```python
from build123d import *

# Parameters (mm, degrees)
F0_W     = 140
F0_H     = 60
F1_DEPTH = 60
F2_R     = 10
F5_DEPTH = 10
F4_R     = 10
F6_DEPTH = 103.2
F3_R     = 10
F7_DEPTH = 10
F8_R     = 5


with BuildPart() as f1:
    # F0 (on Top) → F1 (new body)
    with BuildSketch(Plane.XY):
        Rectangle(F0_W, F0_H)
    extrude(amount=F1_DEPTH)

    # F2 (on face) → F5 (join)
    with BuildSketch(Plane.XY.offset(60)):
        with Locations((-40, 0)):
            Circle(F2_R)
    extrude(amount=F5_DEPTH)

    # F4 (on face) → F6 (cut)
    with BuildSketch(Plane.XY.offset(60)):
        Circle(F4_R)
    extrude(amount=-F6_DEPTH, mode=Mode.SUBTRACT)

    # F3 (on face) → F7 (cut)
    with BuildSketch(Plane.XY.offset(60)):
        with Locations((40, 0)):
            Circle(F3_R)
    extrude(amount=-F7_DEPTH, mode=Mode.SUBTRACT)

    # F8
    f8_edges = [f1.edges().sort_by_distance(p)[0] for p in [
        (0, 30, 60),
        (-70, 0, 60),
        (0, -30, 60),
        (70, 30, 30),
        (-70, 30, 30),
        (0, 30, 0),
        (70, 0, 0),
        (0, -30, 0),
        (-70, 0, 0),
        (70, -30, 30),
    ]]
    fillet(f8_edges, radius=F8_R)


solid = f1.part
```
Can you work these out from the model? Positions are in its coordinate system, mm. A direction names the side the tool comes from. Coordinates: 2 decimals unless noted, no trailing zeros. Loops run counter-clockwise (first coordinate to the right, second up) from the corner with the lowest first, then second, coordinate; pieces in that order, holes last. Notation, with made-up numbers: (76.25, 28) - (84.25, 28) arc R19 ccw to (84.25, 57) - close; hole circle Ø2 at (-37.5, -26.75). An arc over 180 degrees is marked (long way). Answer as CSV lines item,"result". Start each with the question number.
1) I need wall thicknesses on line 1 (X direction, y = 0.5, z = 30); line 2 (Y direction, x = 40, z = 52.5); line 3 (Z direction, x = -33, y = 11). Which ranges of each line are inside material? Lowest first, please. Write a range as from..to.
2) Thinking about a two-plate mould opening in Y: for faces 3 (the cylindrical face through (-69, 28, 30)), 4 (the flat face through (-3, -30, 30)), 5 (the cylindrical face through (30, 0, 55)), which applies, pulls with the +Y half, pulls with the -Y half, needs draft (parallel to the pull), parting line crosses it, or undercut?
3) For pin 1 (16 mm diameter, centred on x = 40, y = 0, fed in from +Z); pin 2 (2 mm diameter, centred on x = 31.5, y = 20, fed in from +Z), each with a flat end and sliding along its axis, tell me the tip position at first contact or that it passes through.
4) Suppose I cut it at C-C (x = 0). Please give me the cut outline in (y, z).
5) Suppose I cut it at A-A (z = 22). Please give me the cut outline in (x, y).
6) Suppose I cut it at B-B (y = 0). Please give me the cut outline in (x, z).
7) Which directions (+Z, -Z, +X, -X, +Y, -Y) give clear straight access to the entire face, cutting with the end or side of a thin tool? Please do faces 1 (the cylindrical face through (3, 29, 58)), 2 (the flat face through (40, 0, 50)).
8) Suppose I cut it at D-D (x = -51.5). Please give me the cut outline in (y, z), plus the area to 3 significant figures.
Check result:
1,line 1,"x = -70..-9.99, 9.99..70"
1,line 2,"y = -30..-10, 10..30"
1,line 3,"z = 0..60"
2,face 3,"pulls with the +Y half"
2,face 4,"pulls with the -Y half"
2,face 5,"undercut"
3,pin 1,"stops at z = 50"
3,pin 2,"stops at z = 60"
4,outline,"(-30, 5) arc R5 ccw to (-25, 0) - (-10, 0) - (-10, 60) - (-25, 60) arc R5 ccw to (-30, 55) - close; (10, 0) - (25, 0) arc R5 ccw to (30, 5) - (30, 55) arc R5 ccw to (25, 60) - (10, 60) - close"
5,outline,"(-70, -30) - (65, -30) arc R5 ccw to (70, -25) - (70, 25) arc R5 ccw to (65, 30) - (-65, 30) arc R5 ccw to (-70, 25) - close; hole circle Ø20 at (0, 0)"
6,outline,"(-70, 5) arc R5 ccw to (-65, 0) - (-10, 0) - (-10, 60) - (-30, 60) - (-30, 70) - (-50, 70) - (-50, 60) - (-65, 60) arc R5 ccw to (-70, 55) - close; (10, 0) - (65, 0) arc R5 ccw to (70, 5) - (70, 60) - (50, 60) - (50, 50) - (30, 50) - (30, 60) - (10, 60) - close"
7,face 1,"+Z, +X, -X, +Y"
7,face 2,"+Z"
8,outline,"(-30, 5) arc R5 ccw to (-25, 0) - (25, 0) arc R5 ccw to (30, 5) - (30, 55) arc R5 ccw to (25, 60) - (-25, 60) arc R5 ccw to (-30, 55) - close"
8,area,"3,580 mm²"
